Geometry check sheet. Reference: drawing and pictorial views, mm from the part's lowest x, y, z. A direction names the side the tool comes from. Round coordinates to 2 decimals unless told otherwise and drop trailing zeros. Write each loop counter-clockwise with the first axis right and the second up, starting at its lowest first coordinate (ties: lowest second). Pieces come first, ordered by that corner, then holes. Notation, with made-up numbers: (-25, 61.25) - (17, 61.25) arc R33 ccw to (17, 97.25) - close; hole circle Ø10 at (-4, 70). An arc over 180 degrees is marked (long way). Return JSON: item names as keys, results as strings.
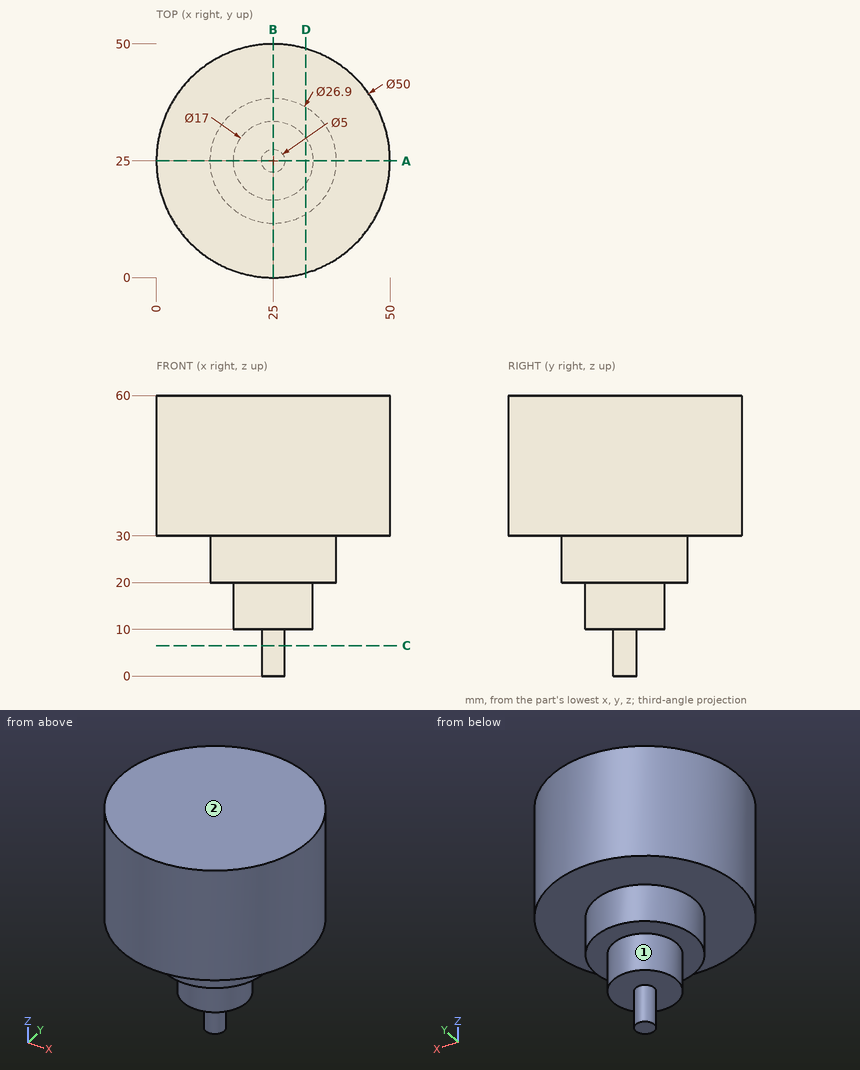
(1) Access from +Z, -Z, +X, -X, +Y, -Y to the whole of each face (thin tool, end or side, straight path). Record for the marked faces 1 and 2.
Response values:
{"face 1": "-Z", "face 2": "+Z, +X, -X, +Y, -Y"}
(2) Gauge pin test, flat ends, axial feed: pin 1 (1.5 mm diameter, centred on y = 39.5, z = 36.5, fed in from -X); pin 2 (2 mm diameter, centred on x = 17, z = 23, fed in from -Y); pin 3 (8 mm diameter, centred on x = 6.5, z = 36.5, fed in from -Y); pin 4 (5 mm diameter, centred on x = 22.5, y = 22.5, fed in from -Z). Record the tip position at first contact, or that the pin passes through.
Response values:
{"pin 1": "stops at x = 4.12", "pin 2": "stops at y = 13.52", "pin 3": "stops at y = 4.63", "pin 4": "stops at z = 0"}
(3) Section check D-D, the plane x = 32. Enter the section's corners in (y, z), plus the area to 3 significant figures.
Response values:
{"outline": "(1, 30) - (13.52, 30) - (13.52, 20) - (20.18, 20) - (20.18, 10) - (29.82, 10) - (29.82, 20) - (36.48, 20) - (36.48, 30) - (49, 30) - (49, 60) - (1, 60) - close", "area": "1,770 mm^2"}
(4) Section check C-C, the plane z = 6.5. Enter the section's corners in (x, y), plus the area to 3 significant figures.
Response values:
{"outline": "circle Ø5 at (25, 25)", "area": "19.6 mm^2"}
(5) Section check A-A, the plane y = 25. Enter the section's corners in (x, z), plus the area to 3 significant figures.
Response values:
{"outline": "(0, 30) - (11.55, 30) - (11.55, 20) - (16.5, 20) - (16.5, 10) - (22.5, 10) - (22.5, 0) - (27.5, 0) - (27.5, 10) - (33.5, 10) - (33.5, 20) - (38.45, 20) - (38.45, 30) - (50, 30) - (50, 60) - (0, 60) - close", "area": "1,990 mm^2"}
(6) Material ranges on line 1 along Z through (x, y) = (19.5, 10.5); line 2 along Z through (x, y) = (22, 21); line 3 along X through (y, z) = (6.5, 44.5), recorded low to high. Write a range as [from, to].
Response values:
{"line 1": "z = [30, 60]", "line 2": "z = [10, 60]", "line 3": "x = [8.18, 41.82]"}
